Model file for the job. Use its own axes, mm. A direction names the side the tool comes from. Give positions to 0.01 mm unless a question says otherwise; leave off trailing zeros. Loops run counter-clockwise (first coordinate to the right, second up) from the corner with the lowest first, then second, coordinate; pieces in that order, holes last. Notation, with made-up numbers: M 14.25,-3 L 56.25,-3 A25 ccw 56.25,9 Z; hole C 31,-18 d4. An arc over 180 degrees is marked long. Answer in a Markdown table with one row per item.
Autodesk Inventor part; units mm, degrees
ref_plane "YZ Plane" through (0, 0, 0) normal (1, 0, 0) x (0, 1, 0)
ref_plane "XZ Plane" through (0, 0, 0) normal (0, 1, 0) x (-1, 0, 0)
ref_plane "XY Plane" through (0, 0, 0) normal (0, 0, 1) x (1, 0, 0)
sketch "Sketch1" plane through (0, 0, 0) normal (0, 0, 1) x (1, 0, 0)
  line L0 (0, 0) -> (-50, 0)
  line L1 (-50, 0) -> (-50, 2)
  line L2 (-46, 4) -> (-46, 2)
  line L3 (-46, 2) -> (-50, 2)
  line L4 (0, 2) -> (-4, 2)
  line L5 (-4, 2) -> (-4, 4)
  line L6 (-46, 4) -> (-26, 4)
  line L7 (0, 2) -> (0, 0)
  line L8 (-26, 4) -> (-26, 2)
  line L9 (-26, 2) -> (-24, 2)
  line L10 (-24, 2) -> (-24, 4)
  line L11 (-24, 4) -> (-4, 4)
  dimension "d2" = 4
  dimension "d3" = 2
  dimension "d5" = 24
  dimension "d6" = 2
  dimension "d7" = 2
extrude "Extrusion1" add sketch "Sketch1" along normal blind 2
sketch "Sketch2" plane through (0, 0, 2) normal (0, 0, 1) x (1, 0, 0)
  line L0 (-4, 4) -> (-24, 4)
  line L1 (-18, 4) -> (-16, 4)
  line L2 (-16, 4) -> (-16, 2)
  line L3 (-16, 2) -> (-18, 2)
  line L4 (-18, 2) -> (-18, 4)
  point P0 (0, 0)
  dimension "d10" = 2
  dimension "d11" = 2
  dimension "d12" = 16
extrude "Extrusion2" cut sketch "Sketch2" against normal blind 2
sketch "Sketch3" plane through (0, 0, 0) normal (0, 0, -1) x (-1, 0, 0)
  line L0 (0, 0) -> (0, 2)
  line L1 (4, 4) -> (16, 4)
  line L2 (0, 0) -> (14, 0)
  line L3 (14, 0) -> (14, 4)
  line L4 (14, 4) -> (0, 4)
  line L5 (0, 4) -> (0, 0)
  line L6 (18, 2) -> (16, 2)
  line L7 (16, 2) -> (14, 2)
  line L8 (14, 2) -> (14, 4)
  line L9 (14, 4) -> (16, 4)
  line L10 (16, 4) -> (16, 2)
  line L11 (18, 4) -> (24, 4)
  line L12 (24, 2) -> (26, 2)
  line L13 (24, 4) -> (26, 4)
  line L14 (26, 4) -> (26, 2)
  line L15 (26, 2) -> (24, 2)
  line L16 (24, 2) -> (24, 4)
  dimension "d15" = 14
extrude "Extrusion3" cut sketch "Sketch3" against normal blind 10 contours L0 L5 L4 L1 L3 L2 | L3 L1 L10 L7
extrude "Extrusion4" add sketch "Sketch3" against normal blind 2 contours L16 L13 L14 L12
properties part number "beam1" material "Wood (Birch)"
Q1. Saw through at C-C (x = -47). Give the cut face in (y, z).
Reported:
| item | result |
|---|---|
| outline | M 0,0 L 2,0 L 2,2 L 0,2 Z |
Q2. Saw through at A-A (z = 1.3). Give the cut face in (x, y).
Reported:
| item | result |
|---|---|
| outline | M -50,0 L -14,0 L -14,2 L -18,2 L -18,4 L -46,4 L -46,2 L -50,2 Z |
Q3. Probe probe 1 along X at (y, z) = (3, 1.8); probe 2 along Y at (x, z) = (-47, 0.5). List the from-to ranges inside material, lowest first.
Reported:
| item | result |
|---|---|
| probe 1 | -46 to -18 |
| probe 2 | 0 to 2 |
Q4. Drop flat-ended pins along their axis: pin 1 (1 mm diameter, centred on y = 3, z = 1, fed in from -X); pin 2 (0.6 mm diameter, centred on x = -15.5, z = 1, fed in from +Y). Give the stop position or say it passes through.
Reported:
| item | result |
|---|---|
| pin 1 | x = -46 |
| pin 2 | y = 2 |
Q5. Saw through at B-B (y = 2.65). Give the cut face in (x, z).
Reported:
| item | result |
|---|---|
| outline | M -46,0 L -18,0 L -18,2 L -46,2 Z |
Q6. 3-axis set-ups, long thin cutter, end or side, ignore diameter. For faces 1 (the face through (-16, 2, 1)), 2 (the face through (-32, 2, 2)), 3 (the face through (-48, 2, 1)): which of +Z, -Z, +X, -X, +Y, -Y reach the whole face in a straight line?
Reported:
| item | result |
|---|---|
| face 1 | +Z, -Z, +X, +Y |
| face 2 | +Z, +X, -X, +Y, -Y |
| face 3 | +Z, -Z, -X, +Y |
